```python
from build123d import *

# Parameters (mm, degrees)
BOSS_EXTRUDE1_DEPTH = 14
SKETCH2_R           = 2.75
CUT_EXTRUDE1_DEPTH  = 14
SKETCH3_R           = 2
CUT_EXTRUDE2_DEPTH  = 45.676615807
SKETCH4_R           = 3.5
CUT_EXTRUDE3_DEPTH  = 3.5
FILLET1_R           = 0.5
CHAMFER1_SIZE       = 0.5


with BuildPart() as part:
    # Sketch1 → Boss-Extrude1 (new body)
    with BuildSketch(Plane(origin=(0, 0, 0), x_dir=(1, 0, 0), z_dir=(0, 1, 0))):
        with BuildLine():
            Line((-21, 3), (-21, -3))
            Line((-21, -3), (21, -3))
            Line((21, -3), (21, 3))
            Line((21, 3), (9, 3))
            Line((9, 3), (9, 30))
            Line((9, 30), (0.75, 30))
            Line((0.75, 30), (0.75, 21.943429983))
            ThreePointArc((0.75, 21.943429983), (0, 12), (-0.75, 21.943429983))
            Line((-0.75, 21.943429983), (-0.75, 30))
            Line((-0.75, 30), (-9, 30))
            Line((-9, 30), (-9, 3))
            Line((-9, 3), (-21, 3))
        make_face()
    extrude(amount=BOSS_EXTRUDE1_DEPTH)

    # Sketch2 → Cut-Extrude1 (cut)
    with BuildSketch(Plane(origin=(0, 0, -3), x_dir=(-1, 0, 0), z_dir=(0, 0, -1))):
        with BuildLine():
            Line((-18.75, 7), (-16, 7))
            Line((-16, 7), (-13.25, 7))
            ThreePointArc((-13.25, 7), (-16, 9.75), (-18.75, 7))
        make_face()
        with BuildLine():
            Line((-13.25, 7), (-16, 7))
            Line((-16, 7), (-18.75, 7))
            ThreePointArc((-18.75, 7), (-16, 4.25), (-13.25, 7))
        make_face()
        with Locations((16, 7)):
            Circle(SKETCH2_R)
    extrude(amount=-CUT_EXTRUDE1_DEPTH, mode=Mode.SUBTRACT)

    # Sketch3 → Cut-Extrude2 (cut, through all)
    with BuildSketch(Plane(origin=(9, 0, 0), x_dir=(0, 0, -1), z_dir=(1, 0, 0))):
        with Locations((24, 7)):
            Circle(SKETCH3_R)
    extrude(amount=-CUT_EXTRUDE2_DEPTH, mode=Mode.SUBTRACT)

    # Sketch4 → Cut-Extrude3 (cut)
    with BuildSketch(Plane(origin=(9, 0, 0), x_dir=(0, 0, -1), z_dir=(1, 0, 0))):
        with Locations((24, 7)):
            Circle(SKETCH4_R)
    extrude(amount=-CUT_EXTRUDE3_DEPTH, mode=Mode.SUBTRACT)

    # Fillet1
    # the kernel refuses this fillet: 0.5 mm, written as the material it adds along each edge
    with BuildSketch(Plane(origin=(9, 0, -3), x_dir=(1, 0, 0), z_dir=(0, 1, 0)), Plane(origin=(-9, 0, -3), x_dir=(0, 0, -1), z_dir=(0, 1, 0))) as fillet1_piece_1:
        with BuildLine():
            CenterArc((FILLET1_R, FILLET1_R), FILLET1_R, 180, 90)
            Line((0, FILLET1_R), (0, 0))
            Line((0, 0), (FILLET1_R, 0))
        make_face()
    extrude(amount=14)
    # the kernel refuses this fillet: 0.5 mm, written as the material it takes off along each edge
    with BuildSketch(Plane(origin=(0.75, -1.031603345, -21.943429983), x_dir=(0.9820189181944738, 0, 0.18878253178765073), z_dir=(0, 1, 0))) as fillet1_2_piece_1:
        with BuildLine():
            CenterArc((0.413109983, 0.499612866), FILLET1_R, 190.881742673, 76.863441213)
            Line((-0.077899477, 0.4052216), (0, 0))
            ThreePointArc((0, 0), (0.196719039, 0.003871337), (0.393438079, 0))
        make_face()
    extrude(amount=16.06320669, mode=Mode.SUBTRACT)
    with BuildSketch(Plane(origin=(0.75, -1.25, -30), x_dir=(0, 0, 1), z_dir=(0, 1, 0))) as fillet1_2_piece_2:
        with BuildLine():
            CenterArc((FILLET1_R, FILLET1_R), FILLET1_R, 180, 90)
            Line((0, FILLET1_R), (0, 0))
            Line((0, 0), (FILLET1_R, 0))
        make_face()
    extrude(amount=16.5, mode=Mode.SUBTRACT)
    with BuildSketch(Plane(origin=(9, -1.25, -30), x_dir=(0, 0, 1), z_dir=(0, 1, 0)), Plane(origin=(-9, -1.25, -30), x_dir=(1, 0, 0), z_dir=(0, 1, 0)), Plane(origin=(-0.75, -1.25, -30), x_dir=(0, 0, 1), z_dir=(0, 1, 0)), Plane(origin=(21, -1.25, 3), x_dir=(-1, 0, 0), z_dir=(0, 1, 0)), Plane(origin=(21, -1.25, -3), x_dir=(0, 0, 1), z_dir=(0, 1, 0)), Plane(origin=(-21, -1.25, -3), x_dir=(1, 0, 0), z_dir=(0, 1, 0)), Plane(origin=(-21, -1.25, 3), x_dir=(0, 0, -1), z_dir=(0, 1, 0))) as fillet1_2_piece_3:
        with BuildLine():
            CenterArc((FILLET1_R, -FILLET1_R), FILLET1_R, 90, 90)
            Line((0, -FILLET1_R), (0, 0))
            Line((0, 0), (FILLET1_R, 0))
        make_face()
    extrude(amount=16.5, mode=Mode.SUBTRACT)
    with BuildSketch(Plane(origin=(-0.75, -1.031603345, -21.943429983), x_dir=(0, 0, -1), z_dir=(0, 1, 0))) as fillet1_2_piece_4:
        with BuildLine():
            CenterArc((0.412641338, 0.5), FILLET1_R, 193.136558787, 76.863441213)
            ThreePointArc((-0.074274237, 0.386363636), (-0.033335392, 0.193912659), (0, 0))
            Line((0, 0), (0.412641338, 0))
        make_face()
    extrude(amount=16.06320669, mode=Mode.SUBTRACT)

    # Chamfer1
    chamfer1_edges = [part.edges().sort_by_distance(p)[0] for p in [
        (-13.25, 7, 3),
        (-13.25, 7, -3),
        (13.25, 7, 3),
        (13.25, 7, -3),
        (-9, 7, -22),
        (9, 7, -20.5),
    ]]
    chamfer(chamfer1_edges, length=CHAMFER1_SIZE)


solid = part.part
```
Input: part model. Units: mm. Frame: model coordinates. A direction names the side the tool comes from. Coordinates: 2 decimals unless noted, no trailing zeros. Write each loop counter-clockwise with the first axis right and the second up, starting at its lowest first coordinate (ties: lowest second). Pieces come first, ordered by that corner, then holes. Notation, with made-up numbers: (70, 82) - (106, 82) arc R11 cw to (106, 97) - close; hole circle Ø10 at (-16.5, -27.75). An arc over 180 degrees is marked (long way). Put each result on its own line as item: value. Start each with the question number.
1) Reachability of faces 4 (the face through (-0.75, 7, -27)), 5 (the face through (9, 7, -16)), 6 (the face through (7.021, 3.895, -25.615)), 7 (the face through (13.818, 8.673, -0.035)) from +Z, -Z, +X, -X, +Y, -Y: full face, straight path, thin tool, end or side. Return the list, or none.
2) Ray query, L1, parallel to Y at x = -4, z = -24; L2, parallel to X at y = 12.5, z = -28; L3, parallel to Z at x = -7, y = 7. Return the intervals inside material, ascending.
3) Cut plane B-B (x = -2). Return the cut outline in (y, z), plus the area to 3 significant figures.
4) Cut plane A-A (z = -17). Return the cut outline in (x, y).
5) Cut plane C-C (x = -16). Return the cut outline in (y, z), plus the area to 3 significant figures.
6) Mould query, pull axis Z, two halves, no side actions, for faces 1 (the face through (3, 7, -22)), 2 (the face through (-9, 7, -17)), 3 (the face through (5, 7, -30)). Classes: pulls with the +Z half, pulls with the -Z half, needs draft (parallel to the pull), parting line crosses it, or undercut.
7) Contact query for flat-ended pins moving along their axis: pin 1 (2 mm diameter, centred on y = 4.5, z = -25.5, fed in from +X); pin 2 (6.5 mm diameter, centred on y = 7, z = -24, fed in from +X); pin 3 (3.5 mm diameter, centred on x = 14, y = 5, fed in from -Z). Output: stop coordinate, or through.
8) Cut plane D-D (z = -24). Return the cut outline in (x, y), plus the area to 3 significant figures.
Resolved:
1. face 4: -Z, +Y, -Y
1. face 5: -Z, +X, +Y, -Y
1. face 6: +X
1. face 7: +Z, -Z
2. L1: y = 0 to 5, 9 to 14
2. L2: x = -9 to -0.75, 0.75 to 9
2. L3: z = -30 to -26, -22 to 3
3. outline: (0, -30) - (14, -30) - (14, -21.58) - (0, -21.58) - close; (0, -12.42) - (14, -12.42) - (14, 3) - (0, 3) - close; hole circle Ø4 at (7, -24)
3. area: 321 mm2
4. outline: (-9, 0) - (-5, 0) - (-5, 14) - (-9, 14) - close; (5, 0) - (9, 0) - (9, 14) - (5, 14) - close
5. outline: (0, -3) - (3.75, -3) - (4.25, -2.5) - (4.25, 2.5) - (3.75, 3) - (0, 3) - close; (9.75, -2.5) - (10.25, -3) - (14, -3) - (14, 3) - (10.25, 3) - (9.75, 2.5) - close
5. area: 50.5 mm2
6. face 1: undercut
6. face 2: needs draft
6. face 3: pulls with the -Z half
7. pin 1: stops at x = 8.92
7. pin 2: stops at x = 5.5
7. pin 3: stops at z = -3
8. outline: (-9, 0) - (-0.75, 0) - (-0.75, 5) - (-8.5, 5) - (-9, 4.5) - close; (-9, 9.5) - (-8.5, 9) - (-0.75, 9) - (-0.75, 14) - (-9, 14) - close; (0.75, 0) - (9, 0) - (9, 3) - (8.5, 3.5) - (5.5, 3.5) - (5.5, 5) - (0.75, 5) - close; (0.75, 9) - (5.5, 9) - (5.5, 10.5) - (8.5, 10.5) - (9, 11) - (9, 14) - (0.75, 14) - close
8. area: 154 mm2
